Autodesk Inventor part; units mm, degrees
ref_plane "YZ Plane" through (0, 0, 0) normal (1, 0, 0) x (0, 1, 0)
ref_plane "XZ Plane" through (0, 0, 0) normal (0, 1, 0) x (-1, 0, 0)
ref_plane "XY Plane" through (0, 0, 0) normal (0, 0, 1) x (1, 0, 0)
sketch "Sketch1" plane through (0, 0, 0) normal (0, 0, 1) x (1, 0, 0)
  line L0 (-17.5, 25) -> (17.5, 25)
  line L1 (17.5, 25) -> (17.5, -25)
  line L2 (17.5, -25) -> (-17.5, -25)
  line L3 (-17.5, -25) -> (-17.5, 25)
  line L4 (17.5, 4.5) -> (12.5, 4.5)
  line L5 (12.5, 4.5) -> (12.5, -4.5)
  line L6 (12.5, -4.5) -> (17.5, -4.5)
  line L7 (17.5, -4.5) -> (17.5, 4.5)
  line L8 (12.5, 12.5) -> (9.5, 12.5)
  line L9 (9.5, 12.5) -> (9.5, -12.5)
  line L10 (9.5, -12.5) -> (12.5, -12.5)
  line L11 (12.5, -12.5) -> (12.5, 12.5)
  point P0 (0, 0)
  point P1 (0, 25)
  point P2 (-17.5, 0)
  point P3 (12.5, 0)
  point P4 (9.5, 0)
  dimension "d0" = 35
  dimension "d1" = 50
  dimension "d7" = 5
  dimension "d8" = 9
  dimension "d9" = 3
  dimension "d10" = 25
extrude "Extrusion1" add sketch "Sketch1" along normal blind 1500 contours L0 L1 L4 L11 L8 L9 L10 L6 L2 L3
fillet "Fillet2" radius 3 10 edges at (17.5, 25, 750) (-17.5, 25, 750) (0, 25, 1500) (-17.5, 0, 1500) (0, -25, 1500) (-17.5, -25, 750) (17.5, -25, 750) (-17.5, 0, 0) (0, 25, 0) (0, -25, 0)
sketch "Sketch3" plane through (-17.5, -22, 3) normal (-1, 0, 0) x (0, 0, 1)
  line L0 (497, 37) -> (997, 37)
  line L1 (997, 37) -> (997, 7)
  line L2 (997, 7) -> (497, 7)
  line L3 (497, 7) -> (497, 37)
  point P0 (-3, 22)
  point P1 (497, 22)
  point P2 (747, 37)
  dimension "d12" = 500
  dimension "d13" = 30
  dimension "d14" = 750
extrude "Extrusion2" add sketch "Sketch3" along normal blind 170
fillet "Fillet3" radius 2 8 edges at (-102.5, -15, 500) (-102.5, 15, 500) (-102.5, 15, 1000) (-102.5, -15, 1000) (-187.5, 15, 750) (-187.5, -15, 750) (-187.5, 0, 500) (-187.5, 0, 1000)
sketch "Sketch4" plane through (-17.5, 15, 998) normal (0, 1, 0) x (1, 0, 0)
  circle A0 centre (-120, 63.5059) radius 17.5
  circle A1 centre (-120, 413.5059) radius 17.5
  line L0 (0, 0) -> (-168, 0)
  line L1 (0, 496) -> (0, 0)
  point P0 (17.5, 998)
  point P1 (-84, 0)
  point P2 (-84, 0)
  dimension "d18" = 35
  dimension "d19" = 35
  dimension "d20" = 350
  dimension "d21" = 73
  dimension "d24" = 120
extrude "Extrusion3" cut sketch "Sketch4" against normal blind 150
properties part number "Soporte Boquillas"
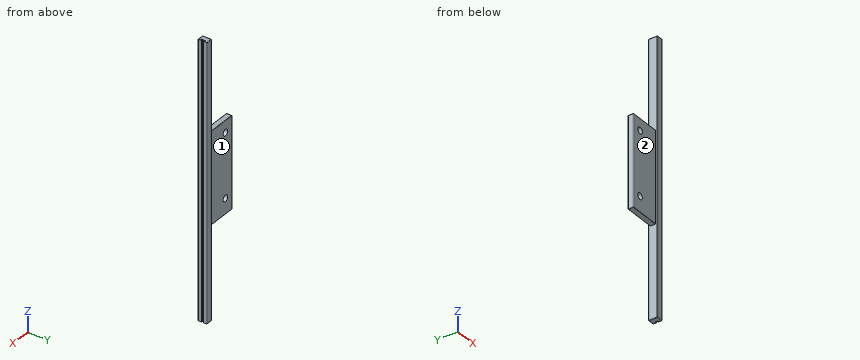
Geometry check sheet. Reference: the model listing, model coordinates, mm. Face numbers are marked on the shaded views. A direction names the side the tool comes from. Round coordinates to 2 decimals unless told otherwise and drop trailing zeros. Write each loop counter-clockwise with the first axis right and the second up, starting at its lowest first coordinate (ties: lowest second). Pieces come first, ordered by that corner, then holes. Notation, with made-up numbers: (3, -6) - (51, -6) arc R25 ccw to (51, 21) - close; hole circle Ø11 at (54, -32). An arc over 180 degrees is marked (long way). One line per item, written item: value.
1. Cross-section at B-B on x = -137.5. Record the boundary of the cut face in (y, z), and give its area (3 significant figures).
The answers:
outline: (-15, 502) arc R2 ccw to (-13, 500) - (13, 500) arc R2 ccw to (15, 502) - (15, 566.99) - (-15, 566.99) - close; (-15, 601.99) - (15, 601.99) - (15, 916.99) - (-15, 916.99) - close; (-15, 951.99) - (15, 951.99) - (15, 998) arc R2 ccw to (13, 1000) - (-13, 1000) arc R2 ccw to (-15, 998) - close
area: 12,900 mm^2
2. Cross-section at C-C on z = 207. Record the boundary of the cut face in (x, y).
The answers:
outline: (-17.5, -22) arc R3 ccw to (-14.5, -25) - (14.5, -25) arc R3 ccw to (17.5, -22) - (17.5, -4.5) - (12.5, -4.5) - (12.5, -12.5) - (9.5, -12.5) - (9.5, 12.5) - (12.5, 12.5) - (12.5, 4.5) - (17.5, 4.5) - (17.5, 22) arc R3 ccw to (14.5, 25) - (-14.5, 25) arc R3 ccw to (-17.5, 22) - close
3. Cross-section at A-A on x = -37. Record the boundary of the cut face in (y, z).
The answers:
outline: (-15, 502) arc R2 ccw to (-13, 500) - (13, 500) arc R2 ccw to (15, 502) - (15, 998) arc R2 ccw to (13, 1000) - (-13, 1000) arc R2 ccw to (-15, 998) - close
4. Scan lines: L1, parallel to Z at x = -137.5, y = 1; L2, parallel to X at y = -11.5, z = 1007; L3, parallel to Z at x = -121.5, y = 13.5. Record each from-to range of solid material in increasing order.
The answers:
L1: z = 500 to 566.99, 601.99 to 916.99, 951.99 to 1000
L2: x = -17.5 to 9.5, 12.5 to 17.5
L3: z = 500.06 to 577.41, 591.58 to 927.41, 941.58 to 999.94
5. Depth check by flat-ended pin: pin 1 Ø13 at (x, y) = (-114.5, 2) entering from +Z; pin 2 Ø1 at (x, z) = (-20.5, 627.5) entering from +Y; pin 3 Ø5 at (x, z) = (-109.5, 498.5) entering from +Y. Enter the tip coordinate at first touch or a pass-through.
The answers:
pin 1: stops at z = 1000
pin 2: stops at y = 15
pin 3: stops at y = 14.73
6. Set-up check for the marked faces 1 and 2: record each of +Z, -Z, +X, -X, +Y, -Y from which the full face is reachable in a straight line by a thin tool's end or side.
The answers:
face 1: +Z, -Z, -X, +Y
face 2: +Z, -Z, -X, -Y
